from build123d import *

# Parameters (mm, degrees)
BOSS_EXTRUDE1_DEPTH = 3.175
SKETCH2_R           = 22.245113978
CUT_EXTRUDE1_DEPTH  = 6.35
EXTRUDE_THIN1_START = 38.35
SKETCH2_2_R         = 25.420113978
SKETCH2_2_R_2       = 22.245113978
EXTRUDE_THIN1_DEPTH = 38.35


with BuildPart() as part:
    # Sketch1 → Boss-Extrude1 (new body)
    with BuildSketch(Plane(origin=(0, 0, 0), x_dir=(1, 0, 0), z_dir=(0, 1, 0))):
        with BuildLine():
            Line((-24.925, 34.925), (24.925, 34.925))
            ThreePointArc((24.925, 34.925), (31.996067812, 31.996067812), (34.925, 24.925))
            Line((34.925, 24.925), (34.925, -24.925))
            ThreePointArc((34.925, -24.925), (31.996067812, -31.996067812), (24.925, -34.925))
            Line((24.925, -34.925), (-24.925, -34.925))
            ThreePointArc((-24.925, -34.925), (-31.996067812, -31.996067812), (-34.925, -24.925))
            Line((-34.925, -24.925), (-34.925, 24.925))
            ThreePointArc((-34.925, 24.925), (-31.996067812, 31.996067812), (-24.925, 34.925))
        make_face()
    extrude(amount=BOSS_EXTRUDE1_DEPTH)

    # Sketch2 → Cut-Extrude1 (cut)
    with BuildSketch(Plane(origin=(0, 3.175, 0), x_dir=(1, 0, 0), z_dir=(0, 1, 0))):
        with Locations(Location((0, 0, 0), (0, 0, 270))):
            Circle(SKETCH2_R)
    extrude(amount=-CUT_EXTRUDE1_DEPTH, mode=Mode.SUBTRACT)

    # Sketch2_2 → Extrude-Thin1 (add)
    with BuildSketch(Plane(origin=(0, 3.175, 0), x_dir=(1, 0, 0), z_dir=(0, 1, 0)).offset(EXTRUDE_THIN1_START)):
        Circle(SKETCH2_2_R)
        Circle(SKETCH2_2_R_2, mode=Mode.SUBTRACT)
    extrude(amount=-EXTRUDE_THIN1_DEPTH)


solid = part.part
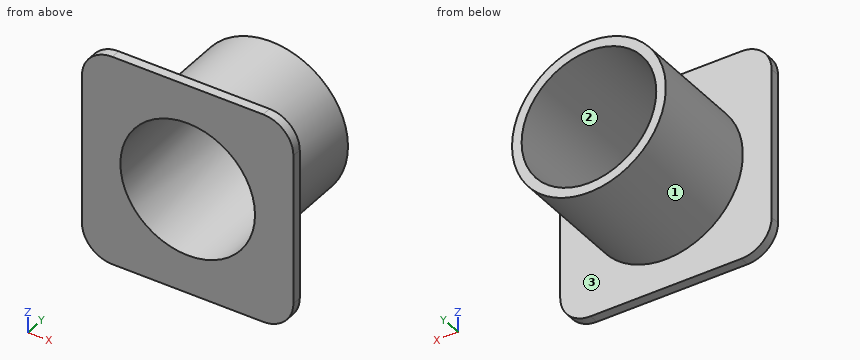
Can you work these out from the model? Positions are in its coordinate system, mm. Face numbers are marked on the shaded views. Round coordinates to 2 decimals unless told otherwise and drop trailing zeros. Write each loop counter-clockwise with the first axis right and the second up, starting at its lowest first coordinate (ties: lowest second). Pieces come first, ordered by that corner, then holes. Notation, with made-up numbers: (72, 26.25) -> (121, 26.25) arc R30 cw to (121, 58.25) -> close; hole circle Ø1 at (-9, -39.75). An arc over 180 degrees is marked (long way). Use one line per item in the form item = value. Start each with the question number.
Q1. Imagine slicing it at A-A (z = -20.5). Please give me the cut outline in (x, y) (3 decimals).
Q2. We'd pull the mould along Z, two halves only. Please class the marked faces 1, 2 and 3: +Z half, -Z half, draft (parallel to the pull), parting line (faces both ways), or undercut.
Q3. Imagine slicing it at B-B (y = 34). Please give me the cut outline in (x, z), then the cut area to 3 significant figures.
Q4. I'm going to push flat-ended pins straight in: P1, Ø2, axis at x = 22, y = 15.5, coming from the +Z side; P2, Ø12, axis at y = 20.5, z = -6, coming from the -X side; P3, Ø10, axis at y = 37, z = 11.5, coming from the +X side. Where does each tip first touch, or does it pass through?
Q5. If I drill on probe 1 along X at (y, z) = (25, 0); probe 2 along Y at (x, z) = (-21.5, 27) (3 decimals), over which ranges is the centre line in solid material (lowest first)? Write a range as [from, to].
Worked out:
q1.outline = (-34.925, 0) -> (-8.637, 0) -> (-8.637, 41.525) -> (-15.031, 41.525) -> (-15.031, 3.175) -> (-34.925, 3.175) -> close; (8.637, 0) -> (34.925, 0) -> (34.925, 3.175) -> (15.031, 3.175) -> (15.031, 41.525) -> (8.637, 41.525) -> close
q2.face_1 = parting line
q2.face_2 = undercut
q2.face_3 = draft
q3.outline = circle Ø50.84 at (0, 0); hole circle Ø44.49 at (0, 0)
q3.area = 475 mm^2
q4.P1 = 14.32
q4.P2 = -25.42
q4.P3 = 24.58
q5.probe_1 = [-25.42, -22.25], [22.25, 25.42]
q5.probe_2 = [0, 3.175]
